For this review, take the finished solid that the model builds, in its own axes (mm). Face numbers are marked on the shaded views. A direction names the side the tool comes from. Round coordinates to 2 decimals unless told otherwise and drop trailing zeros. Order: outer loops, then holes, each group sorted by start corner. A loop starts at its lowest first (then second) coordinate and runs counter-clockwise, first axis right, second up.
from build123d import *

# Parameters (mm, degrees)
SKETCH1_W           = 469
SKETCH1_H           = 1260
BOSS_EXTRUDE1_DEPTH = 779
SKETCH2_W           = 399
SKETCH2_H           = 1190
CUT_EXTRUDE1_DEPTH  = 100
SKETCH3_W           = 1190
SKETCH3_H           = 594
CUT_EXTRUDE3_DEPTH  = 1107.210649018


with BuildPart() as part:
    # Sketch1 → Boss-Extrude1 (new body)
    with BuildSketch(Plane(origin=(0, 0, 0), x_dir=(1, 0, 0), z_dir=(0, 1, 0))):
        Rectangle(SKETCH1_W, SKETCH1_H)
    extrude(amount=-BOSS_EXTRUDE1_DEPTH)

    # Sketch2 → Cut-Extrude1 (cut)
    with BuildSketch(Plane(origin=(0, 0, 0), x_dir=(1, 0, 0), z_dir=(0, 1, 0))):
        Rectangle(SKETCH2_W, SKETCH2_H)
    extrude(amount=-CUT_EXTRUDE1_DEPTH, mode=Mode.SUBTRACT)

    # Sketch3 → Cut-Extrude3 (cut, through all)
    with BuildSketch(Plane.ZY.offset(234.5)):
        with Locations((0, -447)):
            Rectangle(SKETCH3_W, SKETCH3_H)
    extrude(amount=-CUT_EXTRUDE3_DEPTH, mode=Mode.SUBTRACT)


solid = part.part
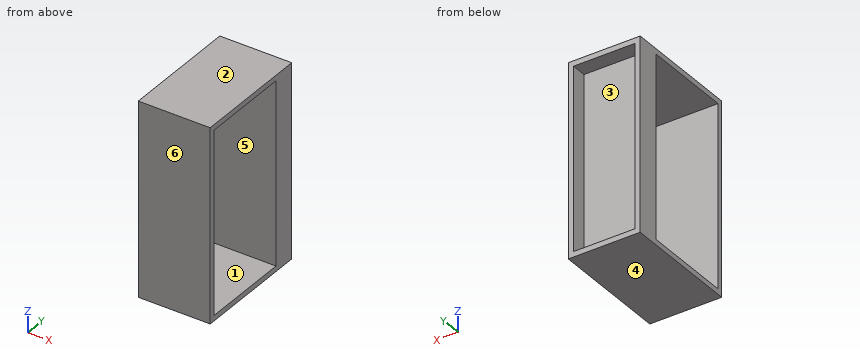
(1) Add section C-C on y = -490. Give the boundary of the cut face in (x, z), plus the area to 3 significant figures.
(2) Draft analysis for pull direction Z (two halves, no side actions). For the marked faces 1, 2, 3 and 4, state which applies: pulls with the +Z half, pulls with the -Z half, needs draft (parallel to the pull), parting line crosses it, or undercut.
(3) Tool access review of the marked faces 5 and 6: name each direction out of +Z, -Z, +X, -X, +Y, -Y from which nothing blocks a thin tool from reaching the whole face with its end or side.
(4) Add section A-A on x = -175. Give the boundary of the cut face in (y, z), plus the area to 3 significant figures.
(5) Clearance check with a flat-ended pin moving along its axis: P1, Ø3, axis at x = -89.5, z = -389, coming from the +Y side. State where the tip first meets the part, or that it passes through.
(6) Add section B-B on z = -151.5. Give the boundary of the cut face in (x, y), plus the area to 3 significant figures.
(7) Wall thickness on L1, parallel to Y at x = -149.5, z = -542; L2, parallel to Z at x = 72, y = -569; L3, parallel to X at y = -61.5, z = -287: over which ranges is each line inside the solid? List them lowest first.
Here are the results:
1. outline: (-234.5, -630) - (234.5, -630) - (234.5, -595) - (-234.5, -595) - close; (-234.5, 595) - (234.5, 595) - (234.5, 630) - (-234.5, 630) - close
1. area: 32,800 mm2
2. face 1: undercut
2. face 2: pulls with the +Z half
2. face 3: undercut
2. face 4: pulls with the -Z half
3. face 5: +X, -X
3. face 6: +Z, -Z, +X, -X, -Y
4. outline: (-779, -630) - (0, -630) - (0, -595) - (-100, -595) - (-100, 595) - (0, 595) - (0, 630) - (-779, 630) - close; hole (-744, -595) - (-150, -595) - (-150, 595) - (-744, 595) - close
4. area: 156,000 mm2
5. P1: stops at y = -100
6. outline: (-234.5, -779) - (234.5, -779) - (234.5, -744) - (-234.5, -744) - close; (-234.5, -150) - (234.5, -150) - (234.5, 0) - (199.5, 0) - (199.5, -100) - (-199.5, -100) - (-199.5, 0) - (-234.5, 0) - close
6. area: 46,900 mm2
7. L1: y = -779 to -744, -150 to -100
7. L2: z = -630 to -595, 595 to 630
7. L3: x = -234.5 to -199.5, 199.5 to 234.5
